Source: CAD feature listing. Evaluate the final solid. Frame: model axes, mm. A direction names the side the tool comes from. Round coordinates to 2 decimals unless told otherwise and drop trailing zeros. Write item = value, one per line. Start each with the question number.
(1) Contact query for flat-ended pins moving along their axis: pin 1 Ø1 at (x, y) = (23.5, -3) entering from +Z; pin 2 Ø4 at (x, z) = (0, -15) entering from -Y; pin 3 Ø6 at (x, z) = (0, 15) entering from -Y; pin 4 Ø2 at (y, z) = (-2.5, -26) entering from +X. Output: stop coordinate, or through.
(2) Cut plane A-A on y = -3.15. Give the number of separate pieces and of enclosed holes in the cut face, then the cut area to 3 significant figures.
(3) Reachability of faces 4 (the face through (35, -2, 0)), 5 (the face through (26.045, -1.972, 15.439)), 6 (the face through (26, -1.972, -15.393)) from +Z, -Z, +X, -X, +Y, -Y: full face, straight path, thin tool, end or side. Return the list, or none.
(4) Draft query along X for faces 1 (the face through (17.36, -2.12, -0.1)), 2 (the face through (-15.393, -1.972, -26)), 3 (the face through (15.439, -1.972, -26.045)). Return one class per face: released by +X, released by -X, zero draft, split by the parting line, or undercut.
(5) Ray query, line 1 (Z direction, x = 0, y = -2.9); line 2 (Z direction, x = 0, y = -0.8); line 3 (Z direction, x = -15, y = -3.4). Return the intervals inside material, ascending.
from build123d import *

# Parameters (mm, degrees)
F0_R           = 35
F0_R_2         = 7.5
F1_DEPTH       = 4
F2_SIZE        = 0.1
F4_D           = 4.5
F4_CSINK_D     = 8.96
F4_CSINK_ANGLE = 90
F6_DEPTH       = 4
F7_R           = 2
F9_D           = 4.2


# Not quite as in the source:
# - a feature names something its author has since deleted; it is built from what else it names


with BuildPart() as f1:
    # F0 (on Front) → F1 (new body)
    with BuildSketch(Plane.XZ):
        Circle(F0_R)
        Circle(F0_R_2, mode=Mode.SUBTRACT)
    extrude(amount=F1_DEPTH)

    # F2
    f2_edges = [f1.edges().sort_by_distance(p)[0] for p in [
        (-35, -4, 0),
        (-35, 0, 0),
        (-7.5, 0, 0),
        (-7.5, -4, 0),
    ]]
    chamfer(f2_edges, length=F2_SIZE)

    # F4 (through all)
    with Locations(Plane(origin=(0, 0, 0), x_dir=(1, 0, 0), z_dir=(0, 1, 0))):
        with Locations((-15, 0), (0, 15), (15, 0), (0, -15)):
            CounterSinkHole(F4_D / 2, F4_CSINK_D / 2, counter_sink_angle=F4_CSINK_ANGLE)

    # F5 (on face) → F6 (cut, through all)
    with BuildSketch(Plane(origin=(0, 0, 0), x_dir=(-1, 0, 0), z_dir=(0, 1, 0))):
        with BuildLine():
            Line((-25.2671224679, -35.8737241857), (-13.7885822331, -24.3951839509))
            ThreePointArc((-13.7885822331, -24.3951839509), (-13.7885822331, -13.7885822331), (-24.3951839509, -13.7885822331))
            Line((-24.3951839509, -13.7885822331), (-35.8737241857, -25.2671224679))
            Line((-35.8737241857, -25.2671224679), (-25.2671224679, -35.8737241857))
        make_face()
        with BuildLine():
            Line((13.7885822331, -24.3951839509), (25.2671224679, -35.8737241857))
            Line((25.2671224679, -35.8737241857), (35.8737241857, -25.2671224679))
            Line((35.8737241857, -25.2671224679), (24.3951839509, -13.7885822331))
            ThreePointArc((24.3951839509, -13.7885822331), (13.7885822331, -13.7885822331), (13.7885822331, -24.3951839509))
        make_face()
        with BuildLine():
            Line((24.3951839509, 13.7885822331), (35.8737241857, 25.2671224679))
            Line((35.8737241857, 25.2671224679), (25.2671224679, 35.8737241857))
            Line((25.2671224679, 35.8737241857), (13.7885822331, 24.3951839509))
            ThreePointArc((13.7885822331, 24.3951839509), (13.7885822331, 13.7885822331), (24.3951839509, 13.7885822331))
        make_face()
        with BuildLine():
            Line((-13.7885822331, 24.3951839509), (-25.2671224679, 35.8737241857))
            Line((-25.2671224679, 35.8737241857), (-35.8737241857, 25.2671224679))
            Line((-35.8737241857, 25.2671224679), (-24.3951839509, 13.7885822331))
            ThreePointArc((-24.3951839509, 13.7885822331), (-13.7885822331, 13.7885822331), (-13.7885822331, 24.3951839509))
        make_face()
    extrude(amount=-F6_DEPTH, mode=Mode.SUBTRACT)

    # F7
    f7_edges = [f1.edges().sort_by_distance(p)[0] for p in [
        (29.47715, -2, -18.870549),
        (18.870549, -2, -29.47715),
        (-18.870549, -2, -29.47715),
        (-29.47715, -2, -18.870549),
        (-29.47715, -2, 18.870549),
        (-18.870549, -2, 29.47715),
        (18.870549, -2, 29.47715),
        (29.47715, -2, 18.870549),
    ]]
    fillet(f7_edges, radius=F7_R)

    # F9 (through all)
    with Locations(Plane.XZ.offset(4)):
        with Locations((0, 28), (28, 0), (0, -28), (-28, 0)):
            Hole(F9_D / 2)


solid = f1.part
Evaluation:
q1.pin_1 = 13.42
q1.pin_2 = through
q1.pin_3 = -4
q1.pin_4 = 16.39
q2.separate_pieces = 1
q2.enclosed_holes = 9
q2.area = 2,720 mm^2
q3.face_4 = +X, +Y, -Y
q3.face_5 = +Z, +Y, -Y
q3.face_6 = -Z, +Y, -Y
q4.face_1 = undercut
q4.face_2 = released by -X
q4.face_3 = released by +X
q5.line_1 = -35 to -30.1, -25.9 to -17.25, -12.75 to -7.5, 7.5 to 12.75, 17.25 to 25.9, 30.1 to 35
q5.line_2 = -35 to -30.1, -25.9 to -18.68, -11.32 to -7.5, 7.5 to 11.32, 18.68 to 25.9, 30.1 to 35
q5.line_3 = -31.62 to -25.61, -12.81 to -2.25, 2.25 to 12.81, 25.61 to 31.62
